Could you check a few things on this model? Use its own coordinates, in mm. Coordinates: 2 decimals unless noted, no trailing zeros. Loops run counter-clockwise (first coordinate to the right, second up) from the corner with the lowest first, then second, coordinate; pieces in that order, holes last. Notation, with made-up numbers: (75, 27.25) - (92, 27.25) arc R25 ccw to (92, 56.25) - close; hole circle Ø1 at (82.25, 26). An arc over 180 degrees is marked (long way). One line per question, with ' | ' between items. Start each with the question number.
1. Please list where these lines run through material, in increasing order: L1, parallel to Y at x = 101.6, z = -11.5; L2, parallel to Y at x = 99.5, z = -20.5; L3, parallel to X at y = 400.5, z = -16. Write a range as [from, to].
2. I'm going to push flat-ended pins straight in: P1, Ø6, axis at y = 361, z = -10.5, coming from the -X side; P2, Ø3, axis at y = 347, z = -17.5, coming from the +X side. Where does each tip first touch, or does it pass through?
3. We'd pull the mould along Y, two halves only. Please class faces 1 (the cylindrical face through (99.366, 419.075, -12.878)), 2 (the flat face through (100, 207, -25.4)), 3 (the cylindrical face through (115.2, 326.1, -12.5)): pulls with the +Y half, pulls with the -Y half, needs draft (parallel to the pull), parting line crosses it, or undercut.
4. I want a section at C-C, the plane z = -12.25. Write out the boundary of the cut face in (x, y).
5. I want a section at D-D, the plane x = 138. Write out the boundary of the cut face in (y, z), then the cut area to 3 significant figures.
6. I want a section at A-A, the plane x = 101.6. Write out the boundary of the cut face in (y, z).
7. I want a section at B-B, the plane y = 304.8. Write out the boundary of the cut face in (x, z), then the cut area to 3 significant figures.
from build123d import *

# Parameters (mm, degrees)
SKETCH1_W           = 203.2
SKETCH1_H           = 25.4
BOSS_EXTRUDE1_DEPTH = 609.6
SKETCH2_R           = 25.273
CUT_EXTRUDE1_DEPTH  = 644.07663618
CUT_EXTRUDE2_DEPTH  = 644.07663618


with BuildPart() as part:
    # Sketch1 → Boss-Extrude1 (new body)
    with BuildSketch(Plane(origin=(0, 0, 0), x_dir=(1, 0, 0), z_dir=(0, 1, 0))):
        with Locations((101.6, 12.7)):
            Rectangle(SKETCH1_W, SKETCH1_H)
    extrude(amount=BOSS_EXTRUDE1_DEPTH)

    # Sketch2 → Cut-Extrude1 (cut, through all)
    with BuildSketch(Plane.XY):
        with Locations((101.6, 304.8)):
            Circle(SKETCH2_R)
    extrude(amount=-CUT_EXTRUDE1_DEPTH, mode=Mode.SUBTRACT)

    # Sketch3 → Cut-Extrude2 (cut, through all)
    with BuildSketch(Plane(origin=(0, 0, -25.4), x_dir=(-1, 0, 0), z_dir=(0, 0, -1))):
        with BuildLine():
            Line((-203.2, 317.5), (-203.2, 609.6))
            Line((-203.2, 609.6), (0, 609.6))
            Line((0, 609.6), (0, 317.5))
            ThreePointArc((0, 317.5), (-101.6, 419.1), (-203.2, 317.5))
        make_face()
    extrude(amount=-CUT_EXTRUDE2_DEPTH, mode=Mode.SUBTRACT)


solid = part.part
Results are:
1) L1: y = [0, 279.53], [330.07, 419.1] | L2: y = [0, 279.61], [329.99, 419.08] | L3: x = [43, 160.2]
2) P1: stops at x = 8.42 | P2: stops at x = 199.27
3) face 1: pulls with the +Y half | face 2: needs draft | face 3: undercut
4) outline: (0, 0) - (203.2, 0) - (203.2, 317.5) arc R101.6 ccw to (0, 317.5) - close; hole circle Ø50.55 at (101.6, 304.8)
5) outline: (0, -25.4) - (412.36, -25.4) - (412.36, 0) - (0, 0) - close | area: 10,500 mm2
6) outline: (0, -25.4) - (279.53, -25.4) - (279.53, 0) - (0, 0) - close; (330.07, -25.4) - (419.1, -25.4) - (419.1, 0) - (330.07, 0) - close
7) outline: (0, -25.4) - (76.33, -25.4) - (76.33, 0) - (0, 0) - close; (126.87, -25.4) - (203.2, -25.4) - (203.2, 0) - (126.87, 0) - close | area: 3,880 mm2
